Read the model definition and answer for the solid it produces. Units are mm, in the model's axes. Give positions to 0.01 mm unless a question says otherwise; leave off trailing zeros. Write each loop counter-clockwise with the first axis right and the second up, starting at its lowest first coordinate (ties: lowest second). Pieces come first, ordered by that corner, then holes. Notation, with made-up numbers: M 20,-22 L 24,-22 A34 ccw 24,11 Z; hole C 34.25,-32.5 d5. An arc over 180 degrees is marked long. Put each result on its own line as item: value.
Autodesk Inventor part; units mm, degrees
ref_plane "YZ Plane" through (0, 0, 0) normal (1, 0, 0) x (0, 1, 0)
ref_plane "XZ Plane" through (0, 0, 0) normal (0, 1, 0) x (-1, 0, 0)
ref_plane "XY Plane" through (0, 0, 0) normal (0, 0, 1) x (1, 0, 0)
sketch "Sketch1" plane through (0, 0, 0) normal (0, 0, 1) x (1, 0, 0)
  line L0 (10, -30) -> (-10, -30)
  line L1 (-10, 30) -> (10, 30)
  line L2 (0, -30) -> (-30, -30)
  line L3 (0, -30) -> (30, -30)
  line L4 (30, -30) -> (30, -10)
  line L5 (-30, -30) -> (-30, -10)
  line L6 (-10, 30) -> (-30, -10)
  line L7 (10, 30) -> (30, -10)
  circle A0 centre (0, 0) radius 2.6
  line L8 (0, 0) -> (0, 20)
  line L9 (0, 0) -> (20, 0) construction
  circle A1 centre (0, 20) radius 2.6
  line L10 (0, 0) -> (0, -20)
  circle A2 centre (0, -20) radius 2.6
  line L11 (0, -20) -> (-20, -20)
  line L12 (0, -20) -> (20, -20) construction
  circle A3 centre (-20, -20) radius 2.6
  circle A4 centre (20, -20) radius 2.6
  dimension "d7" = 60
  dimension "d8" = 5.2
  dimension "d9" = 20
  dimension "d10" = 90
  dimension "d11" = 5.2
  dimension "d12" = 20
  dimension "d13" = 5.2
  dimension "d14" = 20
  dimension "d15" = 180
  dimension "d16" = 5.2
  dimension "d17" = 5.2
extrude "Extrusion1" add sketch "Sketch1" along normal blind 4
properties part number "2020 T Plate Bracket Connectors"
(1) For a pull along X with two mould halves and no side action, classify faces 1 (the face through (0, -6, 0)), 2 (the face through (-0.338, 17.422, 1.972)), 3 (the face through (20, 10, 2)) as +X half, -X half, draft (parallel to the pull), parting line (faces both ways), or undercut.
Result:
face 1: draft
face 2: undercut
face 3: +X half
(2) Section D-D on x = 21 is taken. Determine the outline of the cut face in (y, z).
Result:
outline: M -30,0 L -22.4,0 L -22.4,4 L -30,4 Z; M -17.6,0 L 8,0 L 8,4 L -17.6,4 Z
(3) Straight lines are drawn through the part: line 1 along Y through (x, z) = (0, 1.9); line 2 along Y through (x, z) = (-20, 1.15); line 3 along Y through (x, z) = (22, 3.4). For each, find the intervals that lie inside material, in ascending order. Write a range as from..to.
Result:
line 1: y = -30..-22.6, -17.4..-2.6, 2.6..17.4, 22.6..30
line 2: y = -30..-22.6, -17.4..10
line 3: y = -30..-21.66, -18.34..6
(4) Section A-A on y = 0 is taken. Determine the outline of the cut face in (x, z), and give its area (3 significant figures).
Result:
outline: M -25,0 L -2.6,0 L -2.6,4 L -25,4 Z; M 2.6,0 L 25,0 L 25,4 L 2.6,4 Z
area: 179 mm²
(5) Section B-B on x = 0 is taken. Determine the outline of the cut face in (y, z), and give its area (3 significant figures).
Result:
outline: M -30,0 L -22.6,0 L -22.6,4 L -30,4 Z; M -17.4,0 L -2.6,0 L -2.6,4 L -17.4,4 Z; M 2.6,0 L 17.4,0 L 17.4,4 L 2.6,4 Z; M 22.6,0 L 30,0 L 30,4 L 22.6,4 Z
area: 178 mm²
(6) Section C-C on z = 1 is taken. Determine the outline of the cut face in (x, y), and give its area (3 significant figures).
Result:
outline: M -30,-30 L 30,-30 L 30,-10 L 10,30 L -10,30 L -30,-10 Z; hole C -20,-20 d5.2; hole C 0,-20 d5.2; hole C 0,0 d5.2; hole C 0,20 d5.2; hole C 20,-20 d5.2
area: 2,690 mm²
